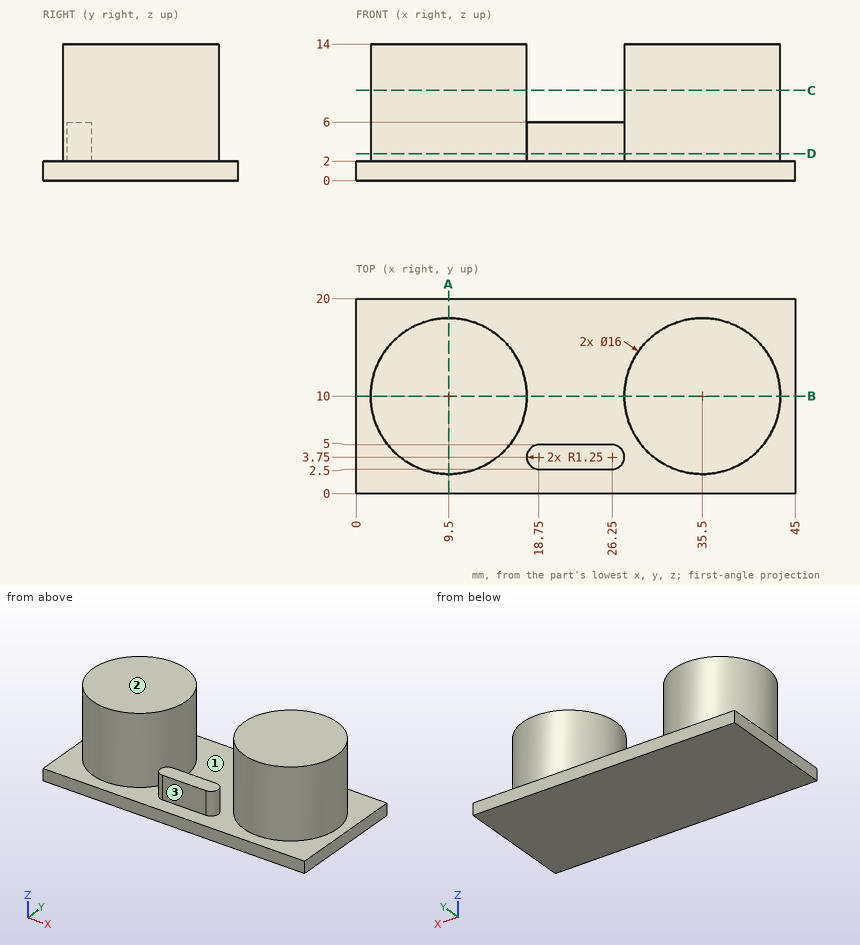
Input: dimensioned drawing with shaded views. Units: mm. Origin: part minimum x, y, z. A direction names the side the tool comes from. Round coordinates to 2 decimals unless told otherwise and drop trailing zeros. Order: outer loops, then holes, each group sorted by start corner. A loop starts at its lowest first (then second) coordinate and runs counter-clockwise, first axis right, second up. Notation, with made-up numbers: (-31.5, 10.25) - (5.5, 10.25) arc R21 ccw to (5.5, 23.25) - close; hole circle Ø2 at (73.25, 25). An arc over 180 degrees is marked (long way). Use CSV: the item, a comma, the result in double quotes. Start each with the question number.
Q1. Section query D-D (z = 2.75). Return loops of the section in (x, y), and give its area (3 significant figures).
Q2. Section query C-C (z = 9.25). Return loops of the section in (x, y), and give its area (3 significant figures).
Q3. Material intervals for line 1 along X through (y, z) = (9.75, 9.75); line 2 along X through (y, z) = (4, 2.5); line 3 along Z through (x, y) = (19, 9), sorted ascending. Write a range as from..to.
Q4. First-contact query: pin 1 (1 mm diameter, centred on x = 12, z = 10.5, fed in from +Y); pin 2 (2 mm diameter, centred on x = 23, y = 4, fed in from +Z); pin 3 (1 mm diameter, centred on y = 16, z = 4, fed in from -X). Flat tips, straight axial feed; report the tip coordinate or a pass-through.
Q5. Access query for the marked faces 1, 2 and 3. Directions: +Z, -Z, +X, -X, +Y, -Y. A direction counts if a zero-diameter tool reaches every point of the face in a straight line with its end or side. Return the directions, or none.
Q6. Section query A-A (x = 9.5). Return loops of the section in (y, z).
Q7. Section query B-B (y = 10). Return loops of the section in (x, z).
Result set:
1,outline,"circle Ø16 at (9.5, 10); (18.75, 2.5) - (26.25, 2.5) arc R1.25 ccw to (26.25, 5) - (18.75, 5) arc R1.25 ccw to start; circle Ø16 at (35.5, 10)"
1,area,"426 mm2"
2,outline,"circle Ø16 at (9.5, 10); circle Ø16 at (35.5, 10)"
2,area,"402 mm2"
3,line 1,"x = 1.5..17.5, 27.5..43.5"
3,line 2,"x = 4.21..14.79, 17.53..27.47, 30.21..40.79"
3,line 3,"z = 0..2"
4,pin 1,"stops at y = 17.75"
4,pin 2,"stops at z = 6"
4,pin 3,"stops at x = 3.69"
5,face 1,"+Z"
5,face 2,"+Z, +X, -X, +Y, -Y"
5,face 3,"+Z, -Y"
6,outline,"(0, 0) - (20, 0) - (20, 2) - (18, 2) - (18, 14) - (2, 14) - (2, 2) - (0, 2) - close"
7,outline,"(0, 0) - (45, 0) - (45, 2) - (43.5, 2) - (43.5, 14) - (27.5, 14) - (27.5, 2) - (17.5, 2) - (17.5, 14) - (1.5, 14) - (1.5, 2) - (0, 2) - close"
